```python
from build123d import *

# Parameters (mm, degrees)
F1_DEPTH = 2210
F2_W     = 340
F2_H     = 940
F3_DEPTH = 400
F4_R     = 77
F5_DEPTH = 25
F6_R     = 77
F7_DEPTH = 25
F8_W     = 200
F8_H     = 250
F9_DEPTH = 10


with BuildPart() as f1:
    # F0 (on Top) → F1 (new body)
    with BuildSketch(Plane.XY):
        Polygon((-830, 0), (0, 0), (0, -700), (100, -700), (100, 500), (-830, 500), align=None)
    extrude(amount=F1_DEPTH)

    # F2 (on face) → F3 (cut)
    with BuildSketch(Plane.XZ):
        with Locations((-170, 1740)):
            Rectangle(F2_W, F2_H)
    extrude(amount=-F3_DEPTH, mode=Mode.SUBTRACT)

    # F4 (on face) → F5 (cut)
    with BuildSketch(Plane.XZ.offset(-400)):
        with Locations((-183, 1532)):
            Circle(F4_R)
    extrude(amount=-F5_DEPTH, mode=Mode.SUBTRACT)

    # F6 (on face) → F7 (cut)
    with BuildSketch(Plane.YZ.offset(-340)):
        with Locations((282, 1862)):
            Circle(F6_R)
    extrude(amount=-F7_DEPTH, mode=Mode.SUBTRACT)

    # F8 (on face) → F9 (join)
    with BuildSketch(Plane.XZ):
        with Locations((-590, 1235)):
            Rectangle(F8_W, F8_H)
    extrude(amount=F9_DEPTH)


solid = f1.part
```
Source: CAD feature listing. Evaluate the final solid. Frame: model axes, mm. A direction names the side the tool comes from. Round coordinates to 2 decimals unless told otherwise and drop trailing zeros. Loops run counter-clockwise (first coordinate to the right, second up) from the corner with the lowest first, then second, coordinate; pieces in that order, holes last.
1. Section query B-B on y = 282. Output: boundary loops of the cut face in (x, z), and give its area (3 significant figures).
2. Contact query for flat-ended pins moving along their axis: pin 1 (6 mm diameter, centred on y = -445.5, z = 386.5, fed in from -X); pin 2 (12 mm diameter, centred on x = -272, z = 802, fed in from -Y); pin 3 (5 mm diameter, centred on x = -564, y = -5.5, fed in from +Z). Output: stop coordinate, or through.
3. Section query C-C on x = -183. Output: boundary loops of the cut face in (y, z), and give its area (3 significant figures).
4. Mould query, pull axis Y, two halves, no side actions, for faces 5 (the cylindrical face through (-352.325, 355.444, 1885.129)), 6 (the flat face through (-172, 197, 1270)), 7 (the flat face through (49, -700, 1090)). Classes: released by +Y, released by -Y, zero draft, split by the parting line, or undercut.
5. Section query D-D on x = -49.5. Output: boundary loops of the cut face in (y, z).
6. Access query for faces 1 (the flat face through (-365, 281, 1863)), 2 (the flat face through (-591, -10, 1237)), 3 (the flat face through (-340, 197, 1733)), 4 (the flat face through (-184, 425, 1533)). Directions: +Z, -Z, +X, -X, +Y, -Y. A direction counts if a zero-diameter tool reaches every point of the face in a straight line with its end or side. Return the directions, or none.
7. Ray query, L1, parallel to Z at x = -183, y = 409.75; L2, parallel to Z at x = -350.5, y = 282; L3, parallel to Y at x = -791, z = 1010.5. Return the intervals inside material, ascending.
8. Section query A-A on z = 1156.5. Output: boundary loops of the cut face in (x, y).
Answers below:
1. outline: (-830, 0) - (100, 0) - (100, 2210) - (0, 2210) - (0, 1270) - (-340, 1270) - (-340, 1785) - (-365, 1785) - (-365, 1939) - (-340, 1939) - (-340, 2210) - (-830, 2210) - close
1. area: 1,730,000 mm2
2. pin 1: stops at x = 0
2. pin 2: stops at y = 0
2. pin 3: stops at z = 1360
3. outline: (0, 0) - (500, 0) - (500, 2210) - (400, 2210) - (400, 1609) - (425, 1609) - (425, 1455) - (400, 1455) - (400, 1270) - (0, 1270) - close
3. area: 725,000 mm2
4. face 5: undercut
4. face 6: zero draft
4. face 7: released by -Y
5. outline: (0, 0) - (500, 0) - (500, 2210) - (400, 2210) - (400, 1270) - (0, 1270) - close
6. face 1: none
6. face 2: +Z, -Z, -X, -Y
6. face 3: +Z, -Y
6. face 4: -Y
7. L1: z = 0 to 1455, 1609 to 2210
7. L2: z = 0 to 1785, 1939 to 2210
7. L3: y = 0 to 500
8. outline: (-830, 0) - (-690, 0) - (-690, -10) - (-490, -10) - (-490, 0) - (0, 0) - (0, -700) - (100, -700) - (100, 500) - (-830, 500) - close
